Print and shaded views of the part. All mm, measured from the part's lowest x, y and z. Coordinates: 2 decimals unless noted, no trailing zeros. Order: outer loops, then holes, each group sorted by start corner. A loop starts at its lowest first (then second) coordinate and runs counter-clockwise, first axis right, second up. Notation, with made-up numbers: (37, -30.5) -> (42, -30.5) arc R30 ccw to (42, -3.5) -> close; hole circle Ø3 at (-34.5, 34). An arc over 180 degrees is marked (long way). Return JSON: item names as keys, results as strings. Group by question number.
1) Cut at C-C (z = 14). Write the cut outline in (x, y), and give its area (3 significant figures).
2) Cut at A-A (x = 23). Write the cut outline in (y, z), and give its area (3 significant figures).
3) Cut at B-B (y = 12). Write the cut outline in (x, z), and give its area (3 significant figures).
4) Cut at D-D (x = 93). Write the cut outline in (y, z).
5) Probe line 1 (Z direction, x = 210, y = 24); line 2 (X direction, y = 5, z = 26.5); line 3 (X direction, y = 9, z = 31) (1 decimal). List the from-to ranges inside material, lowest first.
6) Flat gauge pin, fed straight in: pin 1 (5 mm diameter, centred on x = 206, z = 30.5, fed in from -Y). Where does the tip first touch, or does it go through?
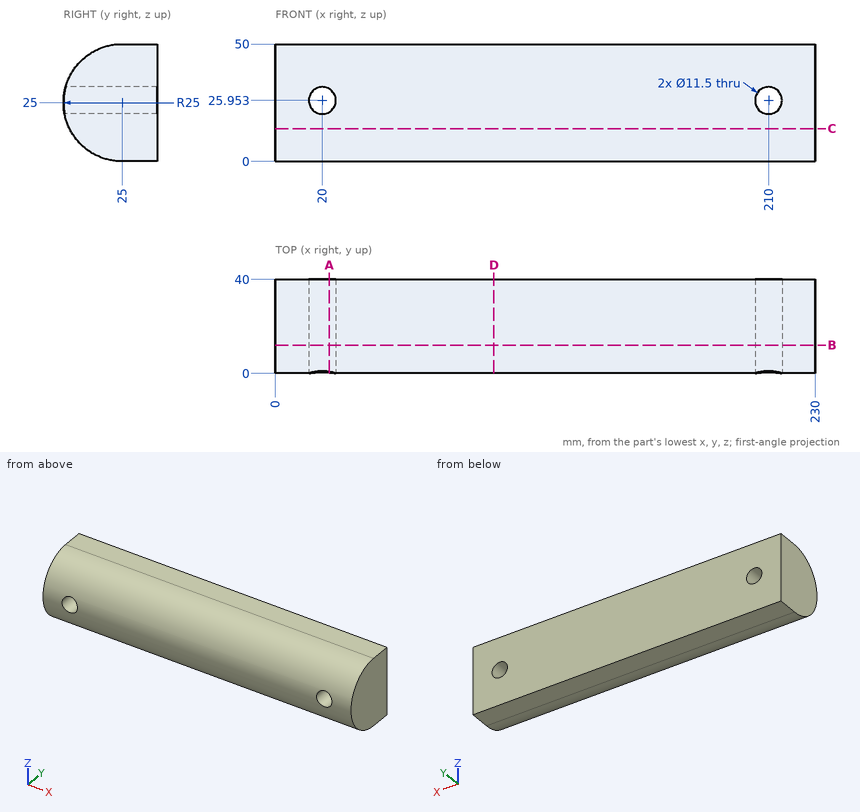
Answers below:
{
 "1": {"outline": "(0, 2.55) -> (230, 2.55) -> (230, 40) -> (0, 40) -> close", "area": "8,610 mm^2"},
 "2": {"outline": "(0.31, 21.05) arc R25 ccw to (25, 0) -> (40, 0) -> (40, 21.05) -> close; (0.7, 30.86) -> (40, 30.86) -> (40, 50) -> (25, 50) arc R25 ccw to start", "area": "1,340 mm^2"},
 "3": {"outline": "(0, 3.65) -> (230, 3.65) -> (230, 46.35) -> (0, 46.35) -> close; hole circle Ø11.5 at (20, 25.95); hole circle Ø11.5 at (210, 25.95)", "area": "9,620 mm^2"},
 "4": {"outline": "(25, 0) -> (40, 0) -> (40, 50) -> (25, 50) arc R25 ccw to start"},
 "5": {"line 1": "z = 0.02 to 20.2, 31.7 to 49.98", "line 2": "x = 0 to 14.28, 25.72 to 204.28, 215.72 to 230", "line 3": "x = 0 to 17.2, 22.8 to 207.2, 212.8 to 230"},
 "6": {"pin 1": "stops at y = 0.22"}
}
